Design review of the part built by this model. Coordinates are the model's own, in mm. Face numbers are marked on the shaded views. A direction names the side the tool comes from. Round coordinates to 2 decimals unless told otherwise and drop trailing zeros. Order: outer loops, then holes, each group sorted by start corner. A loop starts at its lowest first (then second) coordinate and runs counter-clockwise, first axis right, second up. Notation, with made-up numbers: (-10, 57.25) - (21, 57.25) arc R26 cw to (21, 85.25) - close; hole circle Ø11 at (62.25, 7.5). An arc over 180 degrees is marked (long way). Use CSV: the item, a comma, the result in double quotes.
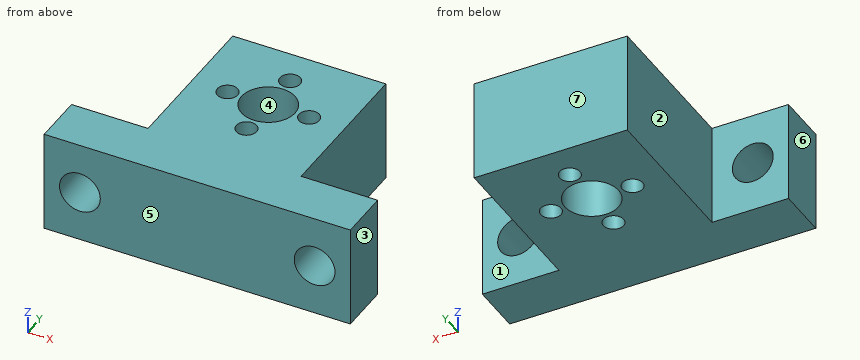
from build123d import *

# Parameters (mm, degrees)
SKETCH1_W           = 60
SKETCH1_H           = 41
SKETCH1_R           = 5.25
SKETCH1_R_2         = 2
BOSS_EXTRUDE1_DEPTH = 20
SKETCH2_R           = 4
CUT_EXTRUDE1_DEPTH  = 42
SKETCH3_W           = 15
SKETCH3_H           = 31
CUT_EXTRUDE2_DEPTH  = 21


with BuildPart() as part:
    # Sketch1 → Boss-Extrude1 (new body)
    with BuildSketch(Plane.XY):
        with Locations((0, -5.5)):
            Rectangle(SKETCH1_W, SKETCH1_H)
        Circle(SKETCH1_R, mode=Mode.SUBTRACT)
        with Locations((0, 8)):
            Circle(SKETCH1_R_2, mode=Mode.SUBTRACT)
        with Locations((8, 0)):
            Circle(SKETCH1_R_2, mode=Mode.SUBTRACT)
        with Locations((0, -8)):
            Circle(SKETCH1_R_2, mode=Mode.SUBTRACT)
        with Locations((-8, 0)):
            Circle(SKETCH1_R_2, mode=Mode.SUBTRACT)
    extrude(amount=BOSS_EXTRUDE1_DEPTH)

    # Sketch2 → Cut-Extrude1 (cut, through all)
    with BuildSketch(Plane(origin=(0, 15, 0), x_dir=(1, 0, 0), z_dir=(0, 1, 0))):
        with Locations((-23, -10)):
            Circle(SKETCH2_R)
        with Locations((23, -10)):
            Circle(SKETCH2_R)
    extrude(amount=-CUT_EXTRUDE1_DEPTH, mode=Mode.SUBTRACT)

    # Sketch3 → Cut-Extrude2 (cut, through all)
    with BuildSketch(Plane(origin=(0, 0, 0), x_dir=(-1, 0, 0), z_dir=(0, 0, -1))):
        with Locations((22.5, -0.5)):
            Rectangle(SKETCH3_W, SKETCH3_H)
        with Locations((-22.5, -0.5)):
            Rectangle(SKETCH3_W, SKETCH3_H)
    extrude(amount=-CUT_EXTRUDE2_DEPTH, mode=Mode.SUBTRACT)


solid = part.part
1) We need section C-C (x = 8). Give the boundary of the cut face in (y, z), then the cut area to 3 significant figures.
Data:
outline,"(-26, 0) - (-2, 0) - (-2, 20) - (-26, 20) - close; (2, 0) - (15, 0) - (15, 20) - (2, 20) - close"
area,"740 mm2"
2) We need section D-D (x = 0). Give the boundary of the cut face in (y, z), then the cut area to 3 significant figures.
Data:
outline,"(-26, 0) - (-10, 0) - (-10, 20) - (-26, 20) - close; (-6, 0) - (-5.25, 0) - (-5.25, 20) - (-6, 20) - close; (5.25, 0) - (6, 0) - (6, 20) - (5.25, 20) - close; (10, 0) - (15, 0) - (15, 20) - (10, 20) - close"
area,"450 mm2"
3) We need section B-B (y = -8). Give the boundary of the cut face in (x, z).
Data:
outline,"(-15, 0) - (-2, 0) - (-2, 20) - (-15, 20) - close; (2, 0) - (15, 0) - (15, 20) - (2, 20) - close"
4) We need section A-A (z = 1.75). Give the boundary of the cut face in (x, y).
Data:
outline,"(-30, -26) - (30, -26) - (30, -16) - (15, -16) - (15, 15) - (-15, 15) - (-15, -16) - (-30, -16) - close; hole circle Ø4 at (-8, 0); hole circle Ø10.5 at (0, 0); hole circle Ø4 at (0, -8); hole circle Ø4 at (0, 8); hole circle Ø4 at (8, 0)"
5) Insertion check: pin 1 Ø4 at (x, y) = (-18.5, -9) entering from -Z; pin 2 Ø4 at (y, z) = (-6.5, 13.5) entering from +X; pin 3 Ø7.5 at (x, z) = (26, 9.5) entering from +Y; pin 4 Ø8 at (y, z) = (-7.5, 4.5) entering from -X. Each pin has a flat end and moves straight along its axis. Give the tip position at first contact, or say it passes through.
Data:
pin 1,"passes through"
pin 2,"stops at x = 15"
pin 3,"stops at y = -16"
pin 4,"stops at x = -15"
6) For the marked faces 1, 2 and 3, list the 3-axis set-ups (+Z, -Z, +X, -X, +Y, -Y) from which the entire face can be reached by the end or side of a thin tool; tool diameter is ignored.
Data:
face 1,"+Z, -Z, +X, +Y"
face 2,"+Z, -Z, -X, +Y"
face 3,"+Z, -Z, +X, +Y, -Y"
7) The part is to be moulded in two halves that separate along Y. For the marked faces 4, 5, 6 and 7, say which applies: +Y half, -Y half, draft (parallel to the pull), parting line (faces both ways), or undercut.
Data:
face 4,"undercut"
face 5,"-Y half"
face 6,"draft"
face 7,"+Y half"
8) To check wall thickness, follow L1, parallel to Y at x = 0, z = 15; L2, parallel to X at y = -21, z = 10; L3, parallel to Y at x = 8, z = 11.25. State the ranges of each line that lie inside material, in increasing order. Write a range as from..to.
Data:
L1,"y = -26..-10, -6..-5.25, 5.25..6, 10..15"
L2,"x = -30..-27, -19..19, 27..30"
L3,"y = -26..-2, 2..15"
